The listing builds one solid part. Answer for the finished solid, in the listing's coordinates (mm). Face numbers are marked on the shaded views. A direction names the side the tool comes from. Round coordinates to 2 decimals unless told otherwise and drop trailing zeros. Order: outer loops, then holes, each group sorted by start corner. A loop starts at its lowest first (then second) coordinate and runs counter-clockwise, first axis right, second up. Notation, with made-up numbers: (84, -26) - (95, -26) arc R20 cw to (95, -14) - close; hole circle Ø4 at (80.25, 26). An arc over 180 degrees is marked (long way). One line per item, written item: value. Start each with the question number.
1. Section C-C, the plane y = -4 is taken. Give the vertices of the cut face in (x, z), then the cut area to 3 significant figures.
2. Section B-B, the plane y = -12.75 is taken. Give the vertices of the cut face in (x, z), then the cut area to 3 significant figures.
3. A tool of negligible diameter and unlimited length cuts with its end or side. For the marked faces 1 and 2, from which of +Z, -Z, +X, -X, +Y, -Y can it reach the whole face along a straight path? Write none if from no direction.
4. Flat-ended cylindrical pins translate along their axes: P1, Ø3, axis at x = 1, y = -10, coming from the +Z side; P2, Ø0.9, axis at x = 5, y = -5, coming from the -Z side. Find the tip coordinate at first contact, or state that the pin passes through.
5. For a pull along Z with two mould halves and no side action, classify the marked faces 3 and 4 as released by +Z, released by -Z, zero draft, split by the parting line, or undercut.
6. Section A-A, the plane z = -25.5 is taken. Give the vertices of the cut face in (x, y).
7. Straight lines are drawn through the part: line 1 (Z direction, x = 2.5, y = -14.3); line 2 (X direction, y = -14.15, z = 25.5); line 3 (Z direction, x = 2.75, y = -7.25). For each, find the intervals that lie inside material, in ascending order.
8. Section D-D, the plane x = 1.6 is taken. Give the vertices of the cut face in (y, z), then the cut area to 3 significant figures.
Autodesk Inventor part; units mm, degrees
ref_plane "YZ Plane" through (0, 0, 0) normal (1, 0, 0) x (0, 1, 0)
ref_plane "XZ Plane" through (0, 0, 0) normal (0, 1, 0) x (-1, 0, 0)
ref_plane "XY Plane" through (0, 0, 0) normal (0, 0, 1) x (1, 0, 0)
sketch "Sketch1" plane through (0, 0, 0) normal (1, 0, 0) x (0, 1, 0)
  line L0 (0, 0) -> (0, 20)
  line L1 (0, 20) -> (-15, 20)
  line L2 (0, 0) -> (3, 0)
  line L3 (3, 0) -> (3, 23)
  line L4 (3, 23) -> (-12, 23)
  line L5 (-12, 23) -> (-12, 28)
  line L6 (-12, 28) -> (-15, 28)
  line L7 (-15, 28) -> (-15, 20)
  line L8 (3.6548, 0) -> (-1.246, 0)
  line L9 (0, 0) -> (0, -20)
  line L10 (0, -20) -> (-15, -20)
  line L11 (3, 0) -> (3, -23)
  line L12 (3, -23) -> (-12, -23)
  line L13 (-12, -23) -> (-12, -28)
  line L14 (-15, -28) -> (-15, -20)
  line L15 (-12, -28) -> (-15, -28)
  dimension "d0" = 20
  dimension "d1" = 15
  dimension "d2" = 3
  dimension "d3" = 23
  dimension "d4" = 15
  dimension "d5" = 5
extrude "Extrusion1" add sketch "Sketch1" along normal blind 5
sketch "Sketch2" plane through (0, -12, 28) normal (0, 1, 0) x (1, 0, 0)
  line L0 (0, 0) -> (0, 2.5)
  line L1 (0, 5) -> (0, 0)
  line L2 (0, 48) -> (0, 56)
  line L3 (0, 56) -> (0, 53.5)
  point P0 (0, 28)
  point P1 (2.5, 2.5)
  point P2 (2.5, 53.5)
  dimension "d8" = 2.5
  dimension "d9" = 2.5
hole "Hole1" at (2.5, -12, 25.5) at (2.5, -12, -25.5) direction (0, -1, 0) diameter 3.4 end through all
sketch "Sketch3" plane through (0, -12, 28) normal (0, 1, 0) x (1, 0, 0)
  circle A0 centre (2.5, 2.5) radius 1.7
  circle A1 centre (2.5, 2.5) radius 3
  circle A2 centre (2.5, 53.5) radius 1.7
  circle A3 centre (2.5, 53.5) radius 3
  point P0 (0, 28)
  dimension "d17" = 6
  dimension "d18" = 6
fillet "Fillet1" radius 2 4 edges at (2.5, 3, 23) (2.5, 0, 20) (2.5, 0, -20) (2.5, 3, -23)
extrude "Extrusion2" cut sketch "Sketch3" along normal blind 20
properties part number "esc-holder"
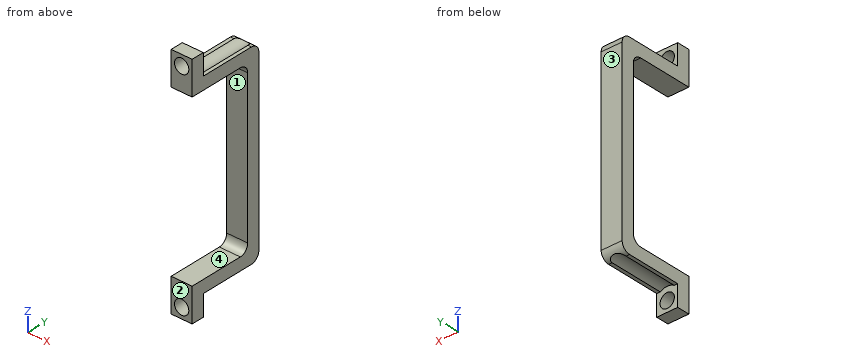
Answer list:
1. outline: (0, -23) - (0.84, -23) arc R3 cw to (4.16, -23) - (5, -23) - (5, -20) - (0, -20) - close; (0, 20) - (5, 20) - (5, 23) - (4.16, 23) arc R3 cw to (0.84, 23) - (0, 23) - close
1. area: 27.7 mm²
2. outline: (0, -28) - (5, -28) - (5, -20) - (0, -20) - close; (0, 20) - (5, 20) - (5, 28) - (0, 28) - close; hole circle Ø3.4 at (2.5, -25.5); hole circle Ø3.4 at (2.5, 25.5)
2. area: 61.8 mm²
3. face 1: +X, -X, -Y
3. face 2: +Z, -Z, +X, -X, -Y
4. P1: stops at z = 23
4. P2: stops at z = -23
5. face 3: zero draft
5. face 4: undercut
6. outline: (0, -15) - (0.8, -15) - (0.8, -12) - (0, -12) - close; (4.2, -15) - (5, -15) - (5, -12) - (4.2, -12) - close
7. line 1: z = -28 to -27.2, -23.8 to -20, 20 to 23.8, 27.2 to 28
7. line 2: x = 0 to 0.8, 4.2 to 5
7. line 3: z = -22.51 to -20, 20 to 22.51
8. outline: (-15, -28) - (-12, -28) - (-12, -26.94) - (-15, -26.94) - close; (-15, -24.06) - (-12, -24.06) - (-12, -22.64) - (2.15, -22.64) arc R2 ccw to (3, -21) - (3, 21) arc R2 ccw to (2.15, 22.64) - (-12, 22.64) - (-12, 24.06) - (-15, 24.06) - (-15, 20) - (-2, 20) arc R2 cw to (0, 18) - (0, -18) arc R2 cw to (-2, -20) - (-15, -20) - close; (-15, 26.94) - (-12, 26.94) - (-12, 28) - (-15, 28) - close
8. area: 231 mm²
